For this review, take the finished solid that the model builds, in its own axes (mm). Face numbers are marked on the shaded views. A direction names the side the tool comes from. Give positions to 0.01 mm unless a question says otherwise; leave off trailing zeros. Order: outer loops, then holes, each group sorted by start corner. A loop starts at its lowest first (then second) coordinate and runs counter-clockwise, first axis right, second up. Notation, with made-up numbers: (63.5, 39.5) -> (74.5, 39.5) arc R27 cw to (74.5, 67.5) -> close; hole circle Ø3 at (20.25, 12). An arc over 180 degrees is marked (long way). Return JSON: item names as keys, results as strings. Group by question number.
1) Add section B-B (x = 0). Give the boundary of the cut face in (y, z), then the cut area to 3 significant figures.
2) For the marked faces 1 and 2, list the 3-axis set-ups (+Z, -Z, +X, -X, +Y, -Y) from which the entire face can be reached by the end or side of a thin tool; tool diameter is ignored.
3) To check wall thickness, follow line 1 along Z through (x, y) = (1.28, 0.2); line 2 along X through (y, z) = (0.5, 8.73); line 3 along Z through (x, y) = (0, 0.8). State the ranges of each line that lie inside material, in increasing order.
4) Add section A-A (z = -7.5). Give the boundary of the cut face in (x, y).
5) Insertion check: P1, Ø1.2, axis at y = -1, z = -1, coming from the -X side; P2, Ø0.8, axis at x = 0.5, y = -1, coming from the -Z side; P3, Ø1.6, axis at x = 1.28, z = 8.73, coming from the -Y side. Each pin has a flat end and moves straight along its axis. Give the tip position at first contact, or say it passes through.
6) Add section D-D (z = 6.21). Give the boundary of the cut face in (x, y), then the cut area to 3 significant figures.
7) Add section C-C (x = -1.28). Give the boundary of the cut face in (y, z), then the cut area to 3 significant figures.
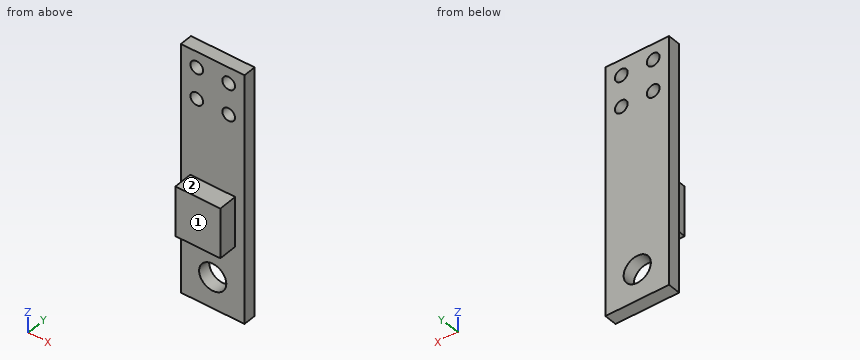
from build123d import *

# Parameters (mm, degrees)
SKETCH1_W    = 5.1
SKETCH1_H    = 20
SKETCH1_R    = 1.09
SKETCH1_R_2  = 0.51
SKETCH1_W_2  = 3.604970558
SKETCH1_H_2  = 4
BODY_DEPTH   = 1.02
SKETCH3_W    = 3.604970558
SKETCH3_H    = 4
SENSOR_DEPTH = 2.52


with BuildPart() as part:
    # Sketch1 → Body (new body)
    with BuildSketch(Plane(origin=(0, 0, 0), x_dir=(1, 0, 0), z_dir=(0, 1, 0))):
        Rectangle(SKETCH1_W, SKETCH1_H)
        with Locations((0, 7.5)):
            Circle(SKETCH1_R, mode=Mode.SUBTRACT)
        with Locations((-1.28, -6.21)):
            Circle(SKETCH1_R_2, mode=Mode.SUBTRACT)
        with Locations((-1.28, -8.73)):
            Circle(SKETCH1_R_2, mode=Mode.SUBTRACT)
        with Locations((1.28, -6.21)):
            Circle(SKETCH1_R_2, mode=Mode.SUBTRACT)
        with Locations((1.28, -8.73)):
            Circle(SKETCH1_R_2, mode=Mode.SUBTRACT)
        with Locations((0, 2.15)):
            Rectangle(SKETCH1_W_2, SKETCH1_H_2, mode=Mode.SUBTRACT)
    extrude(amount=BODY_DEPTH)

    # Sketch3 → Sensor (add)
    with BuildSketch(Plane(origin=(0, 1.02, 0), x_dir=(1, 0, 0), z_dir=(0, 1, 0))):
        with Locations((0, 2.15)):
            Rectangle(SKETCH3_W, SKETCH3_H)
    extrude(amount=-SENSOR_DEPTH)


solid = part.part
Evaluation:
{
 "1": {"outline": "(-1.5, -4.15) -> (0, -4.15) -> (0, -6.41) -> (1.02, -6.41) -> (1.02, 10) -> (0, 10) -> (0, -0.15) -> (-1.5, -0.15) -> close; (0, -10) -> (1.02, -10) -> (1.02, -8.59) -> (0, -8.59) -> close", "area": "24.2 mm^2"},
 "2": {"face 1": "+Z, -Z, +X, -X, -Y", "face 2": "+Z, +X, -X, -Y"},
 "3": {"line 1": "-10 to 5.7, 6.72 to 8.22, 9.24 to 10", "line 2": "-2.55 to -1.79, -0.77 to 0.77, 1.79 to 2.55", "line 3": "-10 to -8.59, -6.41 to 10"},
 "4": {"outline": "(-2.55, 0) -> (-1.09, 0) -> (-1.09, 1.02) -> (-2.55, 1.02) -> close; (1.09, 0) -> (2.55, 0) -> (2.55, 1.02) -> (1.09, 1.02) -> close"},
 "5": {"P1": "x = -1.8", "P2": "z = -4.15", "P3": "y = 0"},
 "6": {"outline": "(-2.55, 0) -> (-1.79, 0) -> (-1.79, 1.02) -> (-2.55, 1.02) -> close; (-0.77, 0) -> (0.77, 0) -> (0.77, 1.02) -> (-0.77, 1.02) -> close; (1.79, 0) -> (2.55, 0) -> (2.55, 1.02) -> (1.79, 1.02) -> close", "area": "3.12 mm^2"},
 "7": {"outline": "(-1.5, -4.15) -> (0, -4.15) -> (0, -10) -> (1.02, -10) -> (1.02, 5.7) -> (0, 5.7) -> (0, -0.15) -> (-1.5, -0.15) -> close; (0, 6.72) -> (1.02, 6.72) -> (1.02, 8.22) -> (0, 8.22) -> close; (0, 9.24) -> (1.02, 9.24) -> (1.02, 10) -> (0, 10) -> close", "area": "24.3 mm^2"}
}
